CAD build for the part. Positions are in the model's coordinates, mm. Give positions to 0.01 mm unless a question says otherwise; leave off trailing zeros. Order: outer loops, then holes, each group sorted by start corner. A loop starts at its lowest first (then second) coordinate and runs counter-clockwise, first axis right, second up. Notation, with made-up numbers: (-10.5, 74) -> (20.5, 74) arc R16 ccw to (20.5, 103) -> close; hole circle Ø6 at (57.5, -22.5). An arc over 180 degrees is marked (long way). Answer as CSV lines item,"result".
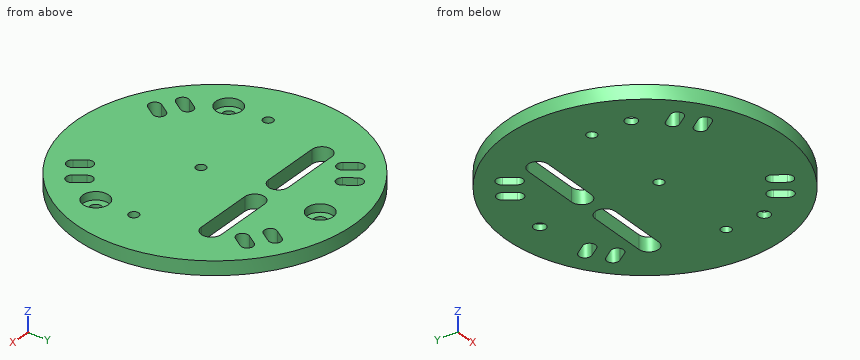
```python
from build123d import *

# Parameters (mm, degrees)
CROQUIS2_R              = 35
SALIENTE_EXTRUIR1_DEPTH = 3.5
CORTAR_EXTRUIR3_DEPTH   = 50.621064076
CORTAR_EXTRUIR4_START   = -3.5
CROQUIS4_R              = 1.25
CORTAR_EXTRUIR4_DEPTH   = 54.121064076
CROQUIS6_R              = 3.25
CORTAR_EXTRUIR6_DEPTH   = 2
CROQUIS7_R              = 1.5
CORTAR_EXTRUIR7_DEPTH   = 50.621064076
CORTAR_EXTRUIR9_DEPTH   = 50.621064076


with BuildPart() as part:
    # Croquis2 → Saliente-Extruir1 (new body)
    with BuildSketch(Plane.XY):
        Circle(CROQUIS2_R)
    extrude(amount=SALIENTE_EXTRUIR1_DEPTH)

    # Croquis3 → Cortar-Extruir3 (cut, through all)
    with BuildSketch(Plane.XY):
        with BuildLine():
            Line((11.226803146, 23.879047115), (12.947532455, 26.336503248))
            ThreePointArc((12.947532455, 26.336503248), (15.036625176, 26.70486666), (15.404988588, 24.615773939))
            Line((15.404988588, 24.615773939), (13.684259279, 22.158317806))
            ThreePointArc((13.684259279, 22.158317806), (11.595166558, 21.789954394), (11.226803146, 23.879047115))
        make_face()
        with BuildLine():
            Line((18.599171544, 18.716859188), (20.319900853, 21.174315321))
            ThreePointArc((20.319900853, 21.174315321), (19.951537442, 23.263408042), (17.862444721, 22.89504463))
            Line((17.862444721, 22.89504463), (16.141715412, 20.437588497))
            ThreePointArc((16.141715412, 20.437588497), (16.510078823, 18.348495776), (18.599171544, 18.716859188))
        make_face()
        with BuildLine():
            Line((18.599171544, -18.716859188), (20.319900853, -21.174315321))
            ThreePointArc((20.319900853, -21.174315321), (19.951537442, -23.263408042), (17.862444721, -22.89504463))
            Line((17.862444721, -22.89504463), (16.141715412, -20.437588497))
            ThreePointArc((16.141715412, -20.437588497), (16.510078823, -18.348495776), (18.599171544, -18.716859188))
        make_face()
        with BuildLine():
            Line((11.226803146, -23.879047115), (12.947532455, -26.336503248))
            ThreePointArc((12.947532455, -26.336503248), (15.036625176, -26.70486666), (15.404988588, -24.615773939))
            Line((15.404988588, -24.615773939), (13.684259279, -22.158317806))
            ThreePointArc((13.684259279, -22.158317806), (11.595166558, -21.789954394), (11.226803146, -23.879047115))
        make_face()
        with BuildLine():
            Line((-11.226803146, -23.879047115), (-12.947532455, -26.336503248))
            ThreePointArc((-12.947532455, -26.336503248), (-15.036625176, -26.70486666), (-15.404988588, -24.615773939))
            Line((-15.404988588, -24.615773939), (-13.684259279, -22.158317806))
            ThreePointArc((-13.684259279, -22.158317806), (-11.595166558, -21.789954394), (-11.226803146, -23.879047115))
        make_face()
        with BuildLine():
            Line((-18.599171544, -18.716859188), (-20.319900853, -21.174315321))
            ThreePointArc((-20.319900853, -21.174315321), (-19.951537442, -23.263408042), (-17.862444721, -22.89504463))
            Line((-17.862444721, -22.89504463), (-16.141715412, -20.437588497))
            ThreePointArc((-16.141715412, -20.437588497), (-16.510078823, -18.348495776), (-18.599171544, -18.716859188))
        make_face()
        with BuildLine():
            Line((-18.599171544, 18.716859188), (-20.319900853, 21.174315321))
            ThreePointArc((-20.319900853, 21.174315321), (-19.951537442, 23.263408042), (-17.862444721, 22.89504463))
            Line((-17.862444721, 22.89504463), (-16.141715412, 20.437588497))
            ThreePointArc((-16.141715412, 20.437588497), (-16.510078823, 18.348495776), (-18.599171544, 18.716859188))
        make_face()
        with BuildLine():
            Line((-11.226803146, 23.879047115), (-12.947532455, 26.336503248))
            ThreePointArc((-12.947532455, 26.336503248), (-15.036625176, 26.70486666), (-15.404988588, 24.615773939))
            Line((-15.404988588, 24.615773939), (-13.684259279, 22.158317806))
            ThreePointArc((-13.684259279, 22.158317806), (-11.595166558, 21.789954394), (-11.226803146, 23.879047115))
        make_face()
    extrude(amount=CORTAR_EXTRUIR3_DEPTH, mode=Mode.SUBTRACT)

    # Croquis4 → Cortar-Extruir4 (cut, through all)
    with BuildSketch(Plane.XY.offset(3.5).offset(CORTAR_EXTRUIR4_START)):
        with Locations((-23.2, -3.5)):
            Circle(CROQUIS4_R)
        with Locations((23.2, -3.5)):
            Circle(CROQUIS4_R)
        with Locations((0, -3.5)):
            Circle(CROQUIS4_R)
    extrude(amount=CORTAR_EXTRUIR4_DEPTH, mode=Mode.SUBTRACT)

    # Croquis6 → Cortar-Extruir6 (cut)
    with BuildSketch(Plane.XY.offset(3.5)):
        with Locations((0, 26.5)):
            Circle(CROQUIS6_R)
        with Locations((22.9496732, -13.25)):
            Circle(CROQUIS6_R)
        with Locations((-22.9496732, -13.25)):
            Circle(CROQUIS6_R)
    extrude(amount=-CORTAR_EXTRUIR6_DEPTH, mode=Mode.SUBTRACT)

    # Croquis7 → Cortar-Extruir7 (cut, through all)
    with BuildSketch(Plane.XY.offset(3.5)):
        with Locations((0, 26.5)):
            Circle(CROQUIS7_R)
        with Locations((22.9496732, -13.25)):
            Circle(CROQUIS7_R)
        with Locations((-22.9496732, -13.25)):
            Circle(CROQUIS7_R)
    extrude(amount=-CORTAR_EXTRUIR7_DEPTH, mode=Mode.SUBTRACT)

    # Croquis10 → Cortar-Extruir9 (cut, through all)
    with BuildSketch(Plane.XY.offset(3.5)):
        with BuildLine():
            Line((-19.1, 15.5), (-4.1, 15.5))
            ThreePointArc((-4.1, 15.5), (-1.6, 13), (-4.1, 10.5))
            Line((-4.1, 10.5), (-19.1, 10.5))
            ThreePointArc((-19.1, 10.5), (-21.6, 13), (-19.1, 15.5))
        make_face()
        with BuildLine():
            Line((19.1, 15.5), (4.1, 15.5))
            ThreePointArc((4.1, 15.5), (1.6, 13), (4.1, 10.5))
            Line((4.1, 10.5), (19.1, 10.5))
            ThreePointArc((19.1, 10.5), (21.6, 13), (19.1, 15.5))
        make_face()
    extrude(amount=-CORTAR_EXTRUIR9_DEPTH, mode=Mode.SUBTRACT)


solid = part.part
```
1) Band-saw the part on D-D, the plane y = -3.5. Write the cut outline in (x, z).
Data:
outline,"(-34.82, 0) -> (-24.45, 0) -> (-24.45, 3.5) -> (-34.82, 3.5) -> close; (-21.95, 0) -> (-1.25, 0) -> (-1.25, 3.5) -> (-21.95, 3.5) -> close; (1.25, 0) -> (21.95, 0) -> (21.95, 3.5) -> (1.25, 3.5) -> close; (24.45, 0) -> (34.82, 0) -> (34.82, 3.5) -> (24.45, 3.5) -> close"
2) Wall check: line 1 along Y through (x, z) = (23.2, 2.7); line 2 along Y through (x, z) = (0, 2.35); line 3 along Y through (x, z) = (-13, 2.3). Give the ranges that are in metal, low to high. Write a range as [from, to].
Data:
line 1,"y = [-26.21, -16.49], [-10.01, -4.75], [-2.25, 26.21]"
line 2,"y = [-35, -4.75], [-2.25, 23.25], [29.75, 35]"
line 3,"y = [-32.5, -26.41], [-21.62, 10.5], [15.5, 21.62], [26.41, 32.5]"
3) Pin check, flat tips, straight feed: P1, Ø3, axis at x = -24, y = -14.5, coming from the +Z side; P2, Ø2.5, axis at x = -22.95, y = -13.25, coming from the -Z side (1 decimal); P3, Ø2, axis at y = 9.5, z = 1.5, coming from the -X side; P4, Ø1, axis at x = 9, z = 2, coming from the -Y side. Stop position of each tip, or through.
Data:
P1,"stops at z = 1.5"
P2,"passes through"
P3,"stops at x = -33.95"
P4,"stops at y = -33.95"
4) Band-saw the part on B-B, the plane y = 13. Write the cut outline in (x, z).
Data:
outline,"(-32.5, 0) -> (-21.6, 0) -> (-21.6, 3.5) -> (-32.5, 3.5) -> close; (-1.6, 0) -> (1.6, 0) -> (1.6, 3.5) -> (-1.6, 3.5) -> close; (21.6, 0) -> (32.5, 0) -> (32.5, 3.5) -> (21.6, 3.5) -> close"
5) Band-saw the part on A-A, the plane x = 0. Write the cut outline in (y, z), then the cut area to 3 significant figures.
Data:
outline,"(-35, 0) -> (-4.75, 0) -> (-4.75, 3.5) -> (-35, 3.5) -> close; (-2.25, 0) -> (25, 0) -> (25, 1.5) -> (23.25, 1.5) -> (23.25, 3.5) -> (-2.25, 3.5) -> close; (28, 0) -> (35, 0) -> (35, 3.5) -> (29.75, 3.5) -> (29.75, 1.5) -> (28, 1.5) -> close"
area,"219 mm2"
6) Band-saw the part on C-C, the plane x = 7. Write the cut outline in (y, z), then the cut area to 3 significant figures.
Data:
outline,"(-34.29, 0) -> (10.5, 0) -> (10.5, 3.5) -> (-34.29, 3.5) -> close; (15.5, 0) -> (34.29, 0) -> (34.29, 3.5) -> (15.5, 3.5) -> close"
area,"223 mm2"
